Design review of the part built by this model. Coordinates are the model's own, in mm. Coordinates: 2 decimals unless noted, no trailing zeros. Order: outer loops, then holes, each group sorted by start corner. A loop starts at its lowest first (then second) coordinate and runs counter-clockwise, first axis right, second up. Notation, with made-up numbers: M 31,-24.75 L 88,-24.75 A5 cw 88,-15.75 Z; hole C -0.5,8.25 d8. An arc over 180 degrees is marked long. Use CSV: the item, a comma, the result in double quotes.
```python
from build123d import *

# Parameters (mm, degrees)
F0_R      = 27.305
F1_DEPTH  = 0.8382
F3_DEPTH  = 25.4
F5_DEPTH  = 25.4
F9_DEPTH  = 0.8382
F10_DEPTH = 17.5768
F11_R     = 7.312924092
F12_R     = 0.6966323576


with BuildPart() as f1:
    # F0 (on Top) → F1 (new body)
    with BuildSketch(Plane.XY):
        Circle(F0_R)
    extrude(amount=F1_DEPTH)

    # F2 (on face) → F3 (cut)
    with BuildSketch(Plane.XY.offset(0.8382)):
        with BuildLine():
            Line((27.305, 0), (-27.305, 0))
            ThreePointArc((-27.305, 0), (0, -27.305), (27.305, 0))
        make_face()
    extrude(amount=-F3_DEPTH, mode=Mode.SUBTRACT)

    # F4 (on face) → F5 (cut)
    with BuildSketch(Plane.XY.offset(0.8382)):
        with BuildLine():
            ThreePointArc((-27.305, 0), (0, 15.5481644558), (27.305, 0))
            ThreePointArc((27.305, 0), (0, 27.305), (-27.305, 0))
        make_face()
    extrude(amount=-F5_DEPTH, mode=Mode.SUBTRACT)

    # F7 (on face) + F6 (on face) → F9 (join)
    with BuildSketch(Plane.XY.offset(0.8382)):
        with BuildLine():
            Line((-1.7974979465, 0), (18.003700975, 0))
            ThreePointArc((18.003700975, 0), (18.4250061935, 1.6697896776), (18.566720813, 3.3860683907))
            ThreePointArc((18.566720813, 3.3860683907), (6.3868228012, 13.7079730699), (-1.7974979465, 0))
        make_face()
    with BuildSketch(Plane.XY.offset(0.8382)):
        with BuildLine():
            Line((18.003700975, 0), (-1.7974979465, 0))
            ThreePointArc((-1.7974979465, 0), (8.1031015143, -7.077550908), (18.003700975, 0))
        make_face()
    extrude(amount=-F9_DEPTH)

    # F8 (on face) → F10 (cut)
    with BuildSketch(Plane.XY.offset(0.8382)):
        with BuildLine():
            ThreePointArc((15.935749386, 0), (16.4593427121, 1.6571771644), (16.6363208264, 3.3860683907))
            ThreePointArc((16.6363208264, 3.3860683907), (6.374210288, 11.7423095885), (0.2704536426, 0))
            Line((0.2704536426, 0), (15.935749386, 0))
        make_face()
        with BuildLine():
            Line((15.935749386, 0), (0.2704536426, 0))
            ThreePointArc((0.2704536426, 0), (8.1031015143, -5.1471509214), (15.935749386, 0))
        make_face()
    extrude(amount=-F10_DEPTH, mode=Mode.SUBTRACT)

    # F11
    f11_edges = [f1.edges().sort_by_distance(p)[0] for p in [
        (18.003701, 0, 0.4191),
    ]]
    fillet(f11_edges, radius=F11_R)

    # F12
    f12_edges = [f1.edges().sort_by_distance(p)[0] for p in [
        (27.305, 0, 0.4191),
    ]]
    fillet(f12_edges, radius=F12_R)


solid = f1.part
```
(1) Add section C-C on x = 12.5. State the section outline as (y, z) points, and give its area (3 significant figures).
The answers:
outline,"M -6.11,0 L -3.93,0 L -3.93,0.84 L -6.11,0.84 Z; M 10.7,0 L 12.98,0 L 12.98,0.84 L 10.7,0.84 Z"
area,"3.74 mm2"
(2) Add section D-D on x = -10. State the section outline as (y, z) points.
The answers:
outline,"M 0,0 L 13.93,0 L 13.93,0.84 L 0,0.84 Z"
(3) Add section B-B on y = 2.75. State the section outline as (x, z) points.
The answers:
outline,"M -25.47,0 L -0.41,0 L -0.41,0.84 L -25.47,0.84 Z; M 16.61,0 L 25.47,0 L 25.47,0.84 L 16.61,0.84 Z"
(4) Wall thickness on probe 1 along X at (y, z) = (-3.75, 0.25); probe 2 along X at (y, z) = (9.5, 0.25); probe 3 along Y at (x, z) = (1, 0.25): over which ranges is each line inside the solid? List them lowest first.
The answers:
probe 1,"x = 0.45 to 3.42, 12.78 to 15.76"
probe 2,"x = -18.64 to 2.15, 14.06 to 18.64"
probe 3,"y = -4.3 to -1.34, 8.11 to 15.53"
